```python
from build123d import *


with BuildPart() as part:
    # Esquisse1 → Base-Révolution (revolve)
    with BuildSketch(Plane(origin=(0, 0, 716.131939029), x_dir=(-1, 0, 0), z_dir=(0, 0, -1)), mode=Mode.PRIVATE) as base_r_volution_sk:
        with BuildLine():
            Line((-2169.949576888, 588.734614361), (-2160.449576888, 588.734614361))
            Line((-2160.449576888, 588.734614361), (-2160.449576888, 615.334513232))
            Line((-2160.449576888, 615.334513232), (-2163.449576888, 615.334513232))
            Line((-2163.449576888, 615.334513232), (-2163.949576888, 614.834513232))
            Line((-2163.949576888, 614.834513232), (-2163.949576888, 605.534359442))
            ThreePointArc((-2163.949576888, 605.534359442), (-2164.249653642, 605.234359452), (-2164.549576849, 605.53451295))
            Line((-2164.549576849, 605.53451295), (-2165.449576888, 605.53451295))
            Line((-2165.449576888, 605.53451295), (-2165.449576888, 591.734359161))
            ThreePointArc((-2165.449576888, 591.734359161), (-2165.749653787, 591.434359171), (-2166.049576849, 591.734512958))
            Line((-2166.049576849, 591.734512958), (-2170.449576888, 591.734512958))
            Line((-2170.449576888, 591.734512958), (-2170.449576888, 589.234614361))
            Line((-2170.449576888, 589.234614361), (-2169.949576888, 588.734614361))
        make_face()
    revolve(base_r_volution_sk.sketch.rotate(Axis((2160.449576888, 588.734614361, 716.131939029), (0, 1, 0)), 90), axis=Axis((2160.449576888, 588.734614361, 716.131939029), (0, 1, 0)))


solid = part.part
```
Read the model definition and answer for the solid it produces. Units are mm, in the model's axes. A direction names the side the tool comes from. Round coordinates to 2 decimals unless told otherwise and drop trailing zeros. Write each loop counter-clockwise with the first axis right and the second up, starting at its lowest first coordinate (ties: lowest second). Pieces come first, ordered by that corner, then holes. Notation, with made-up numbers: (78, 67) - (113, 67) arc R33 ccw to (113, 98) - close; hole circle Ø9 at (-36, 42). An arc over 180 degrees is marked (long way). Use CSV: the item, a comma, the result in double quotes.
Q1. A tool of negligible diameter and unlimited length cuts with its end or side. For faces 1 (the flat face through (2160, 615.335, 716)), 2 (the cylindrical face through (2157.5, 610.12, 714.25)), from which of +Z, -Z, +X, -X, +Y, -Y can it reach the whole face along a straight path? Write none if from no direction.
Values:
face 1,"+Z, -Z, +X, -X, +Y"
face 2,"+Y"
Q2. Find section A-A, the plane y = 602.75. Write down the section's boundary in (x, z).
Values:
outline,"circle Ø10 at (2160.45, 716.13)"
Q3. Find section B-B, the plane y = 608. Write down the section's boundary in (x, z).
Values:
outline,"circle Ø7 at (2160.45, 716.13)"
Q4. Straight lines are drawn through the part: line 1 along Y through (x, z) = (2160.75, 723.75); line 2 along Y through (x, z) = (2164.25, 715.5); line 3 along X through (y, z) = (610, 717). For each, find the intervals that lie inside material, in ascending order.
Values:
line 1,"y = 588.73 to 591.73"
line 2,"y = 588.73 to 605.24"
line 3,"x = 2157.06 to 2163.84"
Q5. Each of these flat-tipped pins is pushed along its axis until it touches: pin 1 Ø8 at (x, z) = (2155, 723.5) entering from +Y; pin 2 Ø6 at (x, y) = (2154, 598.5) entering from -Z; pin 3 Ø4 at (x, y) = (2165, 592.5) entering from -Z. Where does it stop, or does it pass through?
Values:
pin 1,"stops at y = 591.73"
pin 2,"stops at z = 712.51"
pin 3,"stops at z = 706.5"
